from build123d import *

# Parameters (mm, degrees)
F0_W      = 6
F0_H      = 16.8
F1_DEPTH  = 3
F0_W_2    = 5
F0_W_3    = 10
F0_H_2    = 8.8
F0_W_4    = 8
F0_H_3    = 8.4
F2_DEPTH  = 6
F0_W_5    = 15.8
F0_H_4    = 2
F3_DEPTH  = 3.6
F4_DEPTH  = 1
F7_DEPTH  = 1
F8_DEPTH  = 1
F9_W      = 2
F9_H      = 8
F10_DEPTH = 2


# Not quite as in the source:
# - a feature names something its author has since deleted; it is built from what else it names


with BuildPart() as f1:
    # F0 (on Top) → F1 (new body)
    with BuildSketch(Plane.XY):
        with Locations((3, 12.4)):
            Rectangle(F0_W, F0_H)
    extrude(amount=F1_DEPTH)

    # F0 (on Top) → F2 (join)
    with BuildSketch(Plane.XY):
        Polygon((0, 4), (0, 20.8), (0, 24.8), (56, 24.8), (56, 26.8), (48, 26.8), (48, 31.8), (50.6, 31.8), (50.6, 33.8), (48, 33.8), (48, 35.6), (50.6, 35.6), (50.6, 37.6), (46, 37.6), (46, 26.8), (-2, 26.8), (-2, -2), (46, -2), (46, -12.8), (50.6, -12.8), (50.6, -10.8), (48, -10.8), (48, -9), (50.6, -9), (50.6, -7), (48, -7), (48, -2), (56, -2), (56, 0), (0, 0), align=None)
    extrude(amount=F2_DEPTH)



with BuildPart() as f1b:
    # F0 (on Top) → F1, piece 2 (new body)
    with BuildSketch(Plane.XY):
        with Locations((14.5, 12.4)):
            Rectangle(F0_W_2, F0_H)
    extrude(amount=F1_DEPTH)


with BuildPart() as f1c:
    # F0 (on Top) → F1, piece 3 (new body)
    with BuildSketch(Plane.XY):
        with Locations((36.3, 12.4)):
            Rectangle(F0_W_3, F0_H_2)
    extrude(amount=F1_DEPTH)


with BuildPart() as f1d:
    # F0 (on Top) → F1, piece 4 (new body)
    with BuildSketch(Plane.XY):
        with Locations((52, 16.6)):
            Rectangle(F0_W_4, F0_H_3)
    extrude(amount=F1_DEPTH)


with BuildPart() as f2:
    # F0 (on Top) → F2, piece 2 (new body)
    with BuildSketch(Plane.XY):
        Polygon((66.4, 33.8), (66.4, 31.8), (69, 31.8), (69, 26.8), (64, 26.8), (64, 24.8), (69, 24.8), (69, 0), (64, 0), (64, -2), (69, -2), (69, -7), (66.4, -7), (66.4, -9), (69, -9), (69, -10.8), (66.4, -10.8), (66.4, -12.8), (71, -12.8), (71, 37.6), (66.4, 37.6), (66.4, 35.6), (69, 35.6), (69, 33.8), align=None)
    extrude(amount=F2_DEPTH)


with BuildPart() as f1_1:
    add(f1.part)

    add(f2.part)  # F3 merges F2
    # F0 (on Top) → F3 (join)
    with BuildSketch(Plane.XY):
        with Locations((58.5, 36.6)):
            Rectangle(F0_W_5, F0_H_4)
        with Locations((58.5, 32.8)):
            Rectangle(F0_W_5, F0_H_4)
        with Locations((58.5, -8)):
            Rectangle(F0_W_5, F0_H_4)
        with Locations((58.5, -11.8)):
            Rectangle(F0_W_5, F0_H_4)
    extrude(amount=F3_DEPTH)

    # F0 (on Top) → F4 (join)
    with BuildSketch(Plane.XY):
        Polygon((48, 33.8), (50.6, 33.8), (66.4, 33.8), (69, 33.8), (69, 35.6), (66.4, 35.6), (50.6, 35.6), (48, 35.6), align=None)
        Polygon((66.4, -9), (50.6, -9), (48, -9), (48, -10.8), (50.6, -10.8), (66.4, -10.8), (69, -10.8), (69, -9), align=None)
    extrude(amount=F4_DEPTH)

    # F5 (on face) + F6 (on face) → F7 (join)
    with BuildSketch(Plane.XY.offset(6)):
        Polygon((48, 31.8), (50.6, 31.8), (50.6, 33.8), (48, 33.8), (48, 35.6), (50.6, 35.6), (50.6, 37.6), (46, 37.6), (46, 31.8), align=None)
        Polygon((48, -7), (46, -7), (46, -12.8), (50.6, -12.8), (50.6, -10.8), (48, -10.8), (48, -9), (50.6, -9), (50.6, -7), align=None)
    with BuildSketch(Plane.XY.offset(6)):
        Polygon((66.4, 33.8), (66.4, 31.8), (69, 31.8), (71, 31.8), (71, 37.6), (66.4, 37.6), (66.4, 35.6), (69, 35.6), (69, 33.8), align=None)
        Polygon((71, -12.8), (71, -7), (69, -7), (66.4, -7), (66.4, -9), (69, -9), (69, -10.8), (66.4, -10.8), (66.4, -12.8), align=None)
    extrude(amount=F7_DEPTH)


    add(f1b.part)  # F8 merges F1b

    add(f1c.part)  # F8 merges F1c

    add(f1d.part)  # F8 merges F1d
    # F0 (on Top) → F8 (join)
    with BuildSketch(Plane.XY):
        Polygon((0, 4), (0, 20.8), (0, 24.8), (56, 24.8), (56, 26.8), (48, 26.8), (48, 31.8), (50.6, 31.8), (50.6, 33.8), (48, 33.8), (48, 35.6), (50.6, 35.6), (50.6, 37.6), (46, 37.6), (46, 26.8), (-2, 26.8), (-2, -2), (46, -2), (46, -12.8), (50.6, -12.8), (50.6, -10.8), (48, -10.8), (48, -9), (50.6, -9), (50.6, -7), (48, -7), (48, -2), (56, -2), (56, 0), (0, 0), align=None)
        Polygon((66.4, 33.8), (66.4, 31.8), (69, 31.8), (69, 26.8), (64, 26.8), (64, 24.8), (69, 24.8), (69, 0), (64, 0), (64, -2), (69, -2), (69, -7), (66.4, -7), (66.4, -9), (69, -9), (69, -10.8), (66.4, -10.8), (66.4, -12.8), (71, -12.8), (71, 37.6), (66.4, 37.6), (66.4, 35.6), (69, 35.6), (69, 33.8), align=None)
        with Locations((58.5, 36.6)):
            Rectangle(F0_W_5, F0_H_4)
        with Locations((58.5, -11.8)):
            Rectangle(F0_W_5, F0_H_4)
        Polygon((0, 24.8), (0, 20.8), (6, 20.8), (6, 4), (0, 4), (0, 0), (56, 0), (56, -2), (48, -2), (48, -7), (50.6, -7), (66.4, -7), (69, -7), (69, -2), (64, -2), (64, 0), (69, 0), (69, 24.8), (64, 24.8), (64, 26.8), (69, 26.8), (69, 31.8), (66.4, 31.8), (50.6, 31.8), (48, 31.8), (48, 26.8), (56, 26.8), (56, 24.8), align=None)
        with Locations((14.5, 12.4)):
            Rectangle(F0_W_2, F0_H, mode=Mode.SUBTRACT)
        with Locations((36.3, 12.4)):
            Rectangle(F0_W_3, F0_H_2, mode=Mode.SUBTRACT)
        with Locations((52, 16.6)):
            Rectangle(F0_W_4, F0_H_3, mode=Mode.SUBTRACT)
    extrude(amount=F8_DEPTH)

    # F9 (on face) → F10 (cut)
    with BuildSketch(Plane.XY.offset(6)):
        with Locations((-1, 12.4)):
            Rectangle(F9_W, F9_H)
    extrude(amount=-F10_DEPTH, mode=Mode.SUBTRACT)


solid = f1_1.part
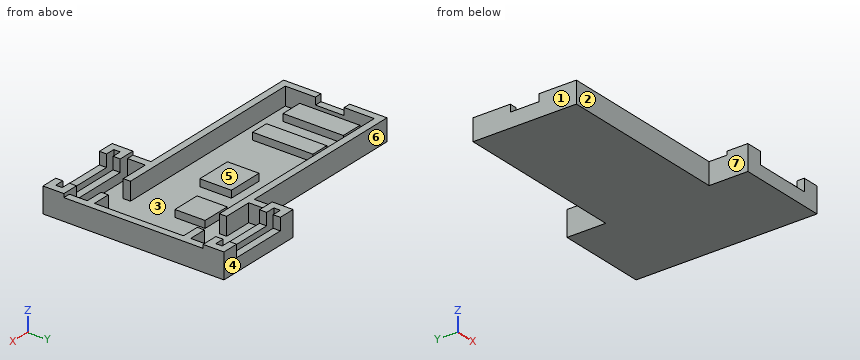
The model under review builds one solid part; all positions refer to its coordinate system, in mm. Face numbers are marked on the shaded views. A direction names the side the tool comes from. Give positions to 0.01 mm unless a question says otherwise; leave off trailing zeros. Order: outer loops, then holes, each group sorted by start corner. A loop starts at its lowest first (then second) coordinate and runs counter-clockwise, first axis right, second up. Notation, with made-up numbers: M 43,19 L 69,19 A35 cw 69,51 Z; hole C 72.5,0.5 d4. An arc over 180 degrees is marked long. Answer in a Markdown table with one row per item. Add a question column.
1. Add section C-C on z = 2. Count the separate pieces of the cut face and the enclosed holes in it, plus the area to 3 significant figures.
2. For pin 1 Ø0.6 at (x, z) = (14.5, 2.5) entering from +Y; pin 2 Ø2.5 at (x, y) = (34.5, 11.5) entering from +Z; pin 3 Ø0.5 at (y, z) = (35, 4.5) entering from -X, all flat-tipped, find the tip position at first contact; note any pin that passes through.
3. Add section A-A on x = 63. State the section outline as (y, z) points, plus the area to 3 significant figures.
4. Add section D-D on x = 13. State the section outline as (y, z) points, plus the area to 3 significant figures.
5. Mouldability with a two-part tool opening along X and no side actions: class the marked faces 1, 2 and 3 as released by +X, released by -X, zero draft, split by the parting line, or undercut.
6. To check wall thickness, follow line 1 along Y through (x, z) = (60, 1.25); line 2 along X through (y, z) = (32, 4.5); line 3 along Y through (x, z) = (31.5, 4). State the ranges of each line that lie inside material, in increasing order.
7. Machinability: for the marked faces 4, 5, 6 and 7, which of the approach directions +Z, -Z, +X, -X, +Y, -Y give a long, thin tool a straight path to every point of the face, cutting with its end or side? Answer none if there is none.
8. Add section B-B on y = 22. State the section outline as (x, z) points, plus the area to 3 significant figures.
The answers:
| question | item | result |
|---|---|---|
| 1 | separate pieces | 4 |
| 1 | enclosed holes | 3 |
| 1 | area | 954 mm2 |
| 2 | pin 1 | y = 26.8 |
| 2 | pin 2 | z = 3 |
| 2 | pin 3 | x = 46 |
| 3 | outline | M -12.8,0 L 37.6,0 L 37.6,3.6 L 35.6,3.6 L 35.6,1 L 33.8,1 L 33.8,3.6 L 31.8,3.6 L 31.8,1 L -7,1 L -7,3.6 L -9,3.6 L -9,1 L -10.8,1 L -10.8,3.6 L -12.8,3.6 Z |
| 3 | area | 71.2 mm2 |
| 4 | outline | M -2,0 L 26.8,0 L 26.8,6 L 24.8,6 L 24.8,1 L 20.8,1 L 20.8,3 L 4,3 L 4,1 L 0,1 L 0,6 L -2,6 Z |
| 4 | area | 82.4 mm2 |
| 5 | face 1 | released by -X |
| 5 | face 2 | zero draft |
| 5 | face 3 | undercut |
| 6 | line 1 | -12.8 to -10.8, -9 to -7, 31.8 to 33.8, 35.6 to 37.6 |
| 6 | line 2 | 46 to 50.6, 66.4 to 71 |
| 6 | line 3 | -2 to 0, 24.8 to 26.8 |
| 7 | face 4 | +Z, -Z, +X, -X, +Y |
| 7 | face 5 | +Z |
| 7 | face 6 | +Z, -Z, -X, +Y |
| 7 | face 7 | +Z, -Z, -X, -Y |
| 8 | outline | M -2,0 L 71,0 L 71,6 L 69,6 L 69,1 L 0,1 L 0,6 L -2,6 Z |
| 8 | area | 93.0 mm2 |
